```python
from build123d import *

# Parameters (mm, degrees)
F0_R     = 11
F1_DEPTH = 18.4658
F2_DEPTH = 5
F3_R     = 8.382
F4_DEPTH = 25.4


# Not quite as in the source:
# - a feature of the source that left no trace in its solid (it failed there, or was rolled back) is left out


with BuildPart() as f1:
    # F0 (on Front) → F1 (new body)
    with BuildSketch(Plane.XZ):
        with BuildLine():
            ThreePointArc((17.9760799845, 15.4450816893), (16.7584308008, 16.7584306274), (15.4450818753, 17.9760798247))
            ThreePointArc((15.4450818753, 17.9760798247), (0, 43.2300002384), (-15.4450818753, 17.9760798247))
            ThreePointArc((-15.4450818753, 17.9760798247), (-16.7584308008, 16.7584306274), (-17.9760799845, 15.4450816893))
            ThreePointArc((-17.9760799845, 15.4450816893), (-43.23, 0), (-17.9760799845, -15.4450816893))
            ThreePointArc((-17.9760799845, -15.4450816893), (-16.7584307141, -16.7584307141), (-15.4450816893, -17.9760799845))
            ThreePointArc((-15.4450816893, -17.9760799845), (0, -43.23), (15.4450816893, -17.9760799845))
            ThreePointArc((15.4450816893, -17.9760799845), (16.7584307141, -16.7584307141), (17.9760799845, -15.4450816893))
            ThreePointArc((17.9760799845, -15.4450816893), (43.23, 0), (17.9760799845, 15.4450816893))
        make_face()
        with Locations((-25.88, 0)):
            Circle(F0_R, mode=Mode.SUBTRACT)
        with Locations((0, -25.88)):
            Circle(F0_R, mode=Mode.SUBTRACT)
        Circle(F0_R, mode=Mode.SUBTRACT)
        with Locations((25.88, 0)):
            Circle(F0_R, mode=Mode.SUBTRACT)
        with Locations((0, 25.88)):
            Circle(F0_R, mode=Mode.SUBTRACT)
    extrude(amount=F1_DEPTH)

    # F0 (on Front) → F2 (join)
    with BuildSketch(Plane.XZ):
        with BuildLine():
            ThreePointArc((17.9760799845, 15.4450816893), (16.7584308008, 16.7584306274), (15.4450818753, 17.9760798247))
            ThreePointArc((15.4450818753, 17.9760798247), (0, 43.2300002384), (-15.4450818753, 17.9760798247))
            ThreePointArc((-15.4450818753, 17.9760798247), (-16.7584308008, 16.7584306274), (-17.9760799845, 15.4450816893))
            ThreePointArc((-17.9760799845, 15.4450816893), (-43.23, 0), (-17.9760799845, -15.4450816893))
            ThreePointArc((-17.9760799845, -15.4450816893), (-16.7584307141, -16.7584307141), (-15.4450816893, -17.9760799845))
            ThreePointArc((-15.4450816893, -17.9760799845), (0, -43.23), (15.4450816893, -17.9760799845))
            ThreePointArc((15.4450816893, -17.9760799845), (16.7584307141, -16.7584307141), (17.9760799845, -15.4450816893))
            ThreePointArc((17.9760799845, -15.4450816893), (43.23, 0), (17.9760799845, 15.4450816893))
        make_face()
        with Locations((-25.88, 0)):
            Circle(F0_R, mode=Mode.SUBTRACT)
        with Locations((0, -25.88)):
            Circle(F0_R, mode=Mode.SUBTRACT)
        Circle(F0_R, mode=Mode.SUBTRACT)
        with Locations((25.88, 0)):
            Circle(F0_R, mode=Mode.SUBTRACT)
        with Locations((0, 25.88)):
            Circle(F0_R, mode=Mode.SUBTRACT)
        with Locations((0, 25.88)):
            Circle(F0_R)
        with Locations((25.88, 0)):
            Circle(F0_R)
        Circle(F0_R)
        with Locations((-25.88, 0)):
            Circle(F0_R)
        with Locations((0, -25.88)):
            Circle(F0_R)
    extrude(amount=-F2_DEPTH)

    # F3 (on face) → F4 (cut)
    with BuildSketch(Plane(origin=(0, 5, 0), x_dir=(-1, 0, 0), z_dir=(0, 1, 0))):
        with Locations((0, 25.88)):
            Circle(F3_R)
        with Locations((-25.88, 0)):
            Circle(F3_R)
        Circle(F3_R)
        with Locations((0, -25.88)):
            Circle(F3_R)
        with Locations((25.88, 0)):
            Circle(F3_R)
    extrude(amount=-F4_DEPTH, mode=Mode.SUBTRACT)


solid = f1.part
```
The model under review builds one solid part; all positions refer to its coordinate system, in mm. A direction names the side the tool comes from. Coordinates: 2 decimals unless noted, no trailing zeros. Write each loop counter-clockwise with the first axis right and the second up, starting at its lowest first coordinate (ties: lowest second). Pieces come first, ordered by that corner, then holes.
1) We need section A-A on x = 25.88. State the section outline as (y, z) points, then the cut area to 3 significant figures.
2) We need section C-C on y = -8.75. State the section outline as (x, z) points.
3) The part is to be moulded in two halves that separate along Z. For faces 1 (the face through (9.4, -18.466, -6.2)), 2 (the face through (43.223, -6.897, -0.496)), 3 (the face through (1.09, 2.54, -17.57)), say which applies: pulls with the +Z half, pulls with the -Z half, needs draft (parallel to the pull), parting line crosses it, or undercut.
4) To check wall thickness, follow probe 1 along Z at (x, y) = (0, 3.4); probe 2 along Z at (x, y) = (0, -9.5); probe 3 along Z at (x, y) = (-25.88, 2.15). State the ranges of each line that lie inside material, in increasing order.
5) Clearance check with flat-ended pins moving along their axes: pin 1 Ø6 at (x, y) = (23.5, -2) entering from +Z; pin 2 Ø4 at (y, z) = (-7, -6.5) entering from +X; pin 3 Ø10 at (x, y) = (16.5, -6.5) entering from +Z. State where each tip first meets the part, or that it passes through.
6) We need section B-B on z = -25.88. State the section outline as (x, y) points.
7) We need section D-D on x = 0. State the section outline as (y, z) points.
8) Machinability: for faces 4 (the face through (9, 5, 1)), 5 (the face through (-16.741, -6.897, 16.776)), 6 (the face through (-36.87, -9.1, 0.48)), which of the approach directions +Z, -Z, +X, -X, +Y, -Y give a long, thin tool a straight path to every point of the face, cutting with its end or side? Answer none if there is none.
Answer list:
1. outline: (-18.47, -17.35) - (5, -17.35) - (5, -8.38) - (0, -8.38) - (0, -11) - (-18.47, -11) - close; (-18.47, 11) - (0, 11) - (0, 8.38) - (5, 8.38) - (5, 17.35) - (-18.47, 17.35) - close
1. area: 324 mm2
2. outline: (-17.98, -15.45) arc R23.7 ccw to (-15.45, -17.98) arc R17.35 ccw (long way) to (15.45, -17.98) arc R23.7 ccw to (17.98, -15.45) arc R17.35 ccw (long way) to (17.98, 15.45) arc R23.7 ccw to (15.45, 17.98) arc R17.35 ccw (long way) to (-15.45, 17.98) arc R23.7 ccw to (-17.98, 15.45) arc R17.35 ccw (long way) to start; hole circle Ø22 at (-25.88, 0); hole circle Ø22 at (0, -25.88); hole circle Ø22 at (0, 0); hole circle Ø22 at (0, 25.88); hole circle Ø22 at (25.88, 0)
3. face 1: needs draft
3. face 2: parting line crosses it
3. face 3: undercut
4. probe 1: z = -43.23 to -34.26, -17.5 to -8.38, 8.38 to 17.5, 34.26 to 43.23
4. probe 2: z = -43.23 to -36.88, -14.88 to -11, 11 to 14.88, 36.88 to 43.23
4. probe 3: z = -17.35 to -8.38, 8.38 to 17.35
5. pin 1: stops at z = 17.35
5. pin 2: stops at x = 42.64
5. pin 3: stops at z = 38.87
6. outline: (-17.35, -18.47) - (-11, -18.47) - (-11, 0) - (-8.38, 0) - (-8.38, 5) - (-17.35, 5) - close; (8.38, 0) - (11, 0) - (11, -18.47) - (17.35, -18.47) - (17.35, 5) - (8.38, 5) - close
7. outline: (-18.47, -43.23) - (5, -43.23) - (5, -34.26) - (0, -34.26) - (0, -36.88) - (-18.47, -36.88) - close; (-18.47, -14.88) - (0, -14.88) - (0, -17.5) - (5, -17.5) - (5, -8.38) - (0, -8.38) - (0, -11) - (-18.47, -11) - close; (-18.47, 11) - (0, 11) - (0, 8.38) - (5, 8.38) - (5, 17.5) - (0, 17.5) - (0, 14.88) - (-18.47, 14.88) - close; (-18.47, 36.88) - (0, 36.88) - (0, 34.26) - (5, 34.26) - (5, 43.23) - (-18.47, 43.23) - close
8. face 4: +Z, -Z, +X, -X, +Y
8. face 5: +Y, -Y
8. face 6: -Y
